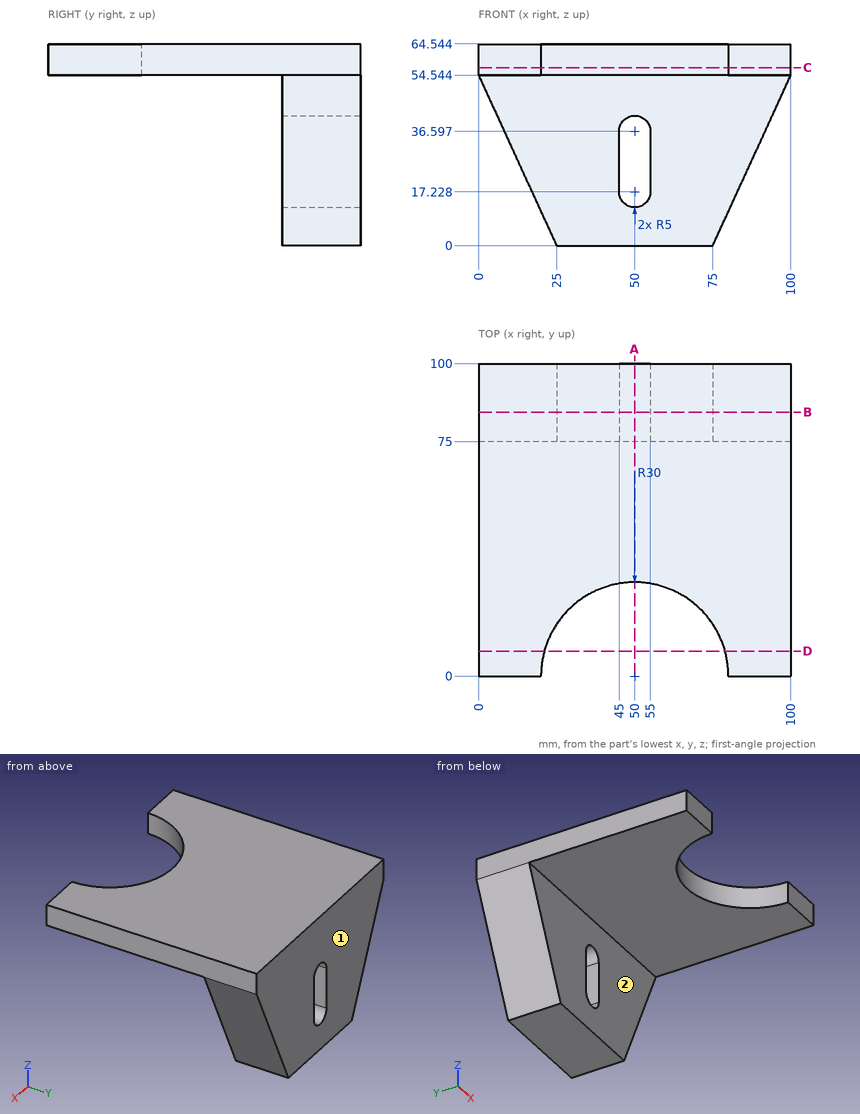
Geometry check sheet. Reference: drawing and pictorial views, mm from the part's lowest x, y, z. A direction names the side the tool comes from. Give positions to 0.01 mm unless a question says otherwise; leave off trailing zeros. Write each loop counter-clockwise with the first axis right and the second up, starting at its lowest first coordinate (ties: lowest second). Pieces come first, ordered by that corner, then holes.
Item 1: Cross-section at A-A (x = 50). Enter the section's corners in (y, z), and give its area (3 significant figures).
Item 2: Cross-section at C-C (z = 57). Enter the section's corners in (x, y).
Item 3: Scan lines: L1, parallel to Y at x = 11, z = 51; L2, parallel to Z at x = 90, y = 42; L3, parallel to X at y = 93, z = 36.5. Record each from-to range of solid material in increasing order.
Item 4: Cross-section at D-D (y = 8). Enter the section's corners in (x, z).
Item 5: Cross-section at B-B (y = 84.5). Enter the section's corners in (x, z).
Item 6: Access from +Z, -Z, +X, -X, +Y, -Y to the whole of each face (thin tool, end or side, straight path). Record for the marked faces 1 and 2.
Item 7: Gauge pin test, flat ends, axial feed: pin 1 (1.5 mm diameter, centred on x = 29.5, z = 14, fed in from -Y); pin 2 (21.5 mm diameter, centred on y = 85.5, z = 26, fed in from +X) (1 decimal); pin 3 (9.5 mm diameter, centred on y = 90.5, z = 28, fed in from -X). Record the tip position at first contact, or that the pin passes through.
Report:
1. outline: (30, 54.54) - (75, 54.54) - (75, 41.6) - (100, 41.6) - (100, 64.54) - (30, 64.54) - close; (75, 0) - (100, 0) - (100, 12.23) - (75, 12.23) - close
1. area: 1,330 mm2
2. outline: (0, 0) - (20, 0) arc R30 cw to (80, 0) - (100, 0) - (100, 100) - (0, 100) - close
3. L1: y = 75 to 100
3. L2: z = 54.54 to 64.54
3. L3: x = 8.27 to 45, 55 to 91.73
4. outline: (0, 54.54) - (21.09, 54.54) - (21.09, 64.54) - (0, 64.54) - close; (78.91, 54.54) - (100, 54.54) - (100, 64.54) - (78.91, 64.54) - close
5. outline: (0, 54.54) - (25, 0) - (75, 0) - (100, 54.54) - (100, 64.54) - (0, 64.54) - close; hole (45, 17.23) arc R5 ccw to (55, 17.23) - (55, 36.6) arc R5 ccw to (45, 36.6) - close
6. face 1: +Z, -Z, +X, -X, +Y
6. face 2: -Z, +X, -X, -Y
7. pin 1: stops at y = 75
7. pin 2: stops at x = 91.8
7. pin 3: stops at x = 9.99
